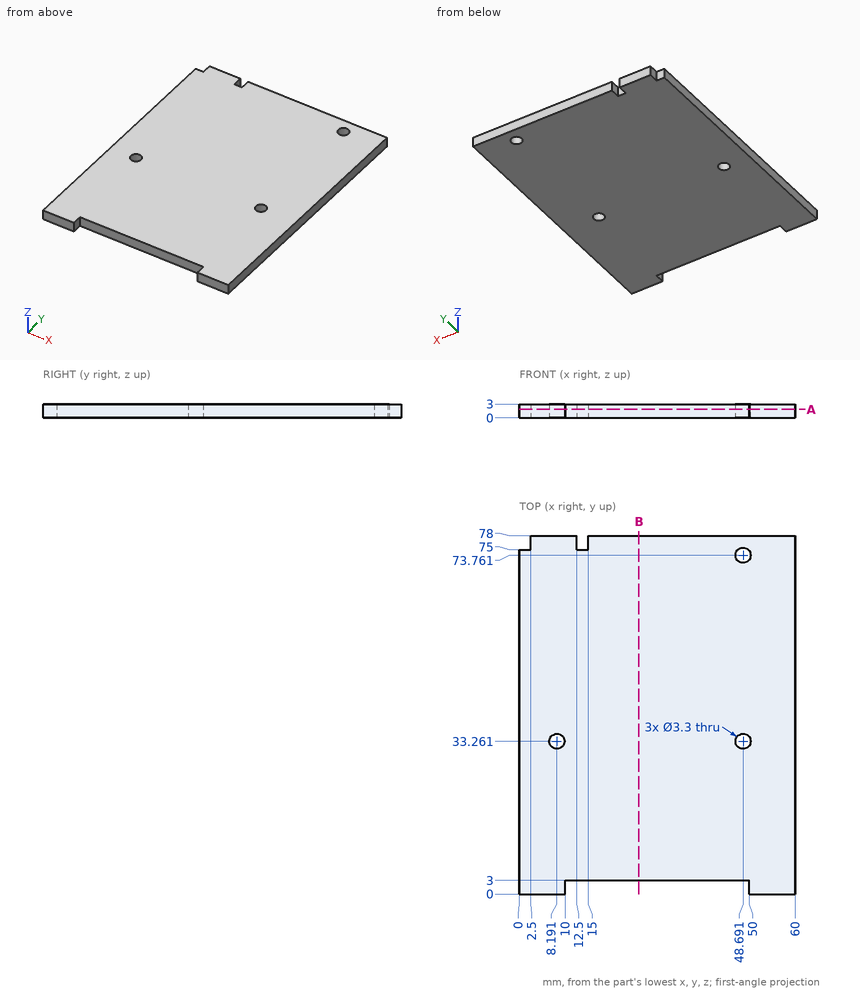
Job drawing, mm, ordinate dimensions from the low corner. One solid piece. Round coordinates to 2 decimals unless told otherwise and drop trailing zeros. Loops run counter-clockwise (first coordinate to the right, second up) from the corner with the lowest first, then second, coordinate; pieces in that order, holes last. Notation, with made-up numbers: (75, 19.5) -> (101, 19.5) arc R8 cw to (101, 33.5) -> close; hole circle Ø5 at (-21.5, 19.5). An arc over 180 degrees is marked (long way). One line per item, written item: value. Start each with the question number.
Q1. Cut at B-B on x = 26. List the corners of the cut face in (y, z).
Q2. Cut at A-A on z = 1.85. List the corners of the cut face in (x, y), plus the area to 3 significant figures.
Q3. Drop flat-ended pins along their axis: pin 1 Ø0.9 at (y, z) = (77, 1.5) entering from -X; pin 2 Ø1 at (y, z) = (30.5, 1.5) entering from -X; pin 3 Ø1.5 at (x, z) = (27, 2) entering from -Y; pin 4 Ø0.8 at (x, z) = (14, 1) entering from +Y. Give the stop position or say it passes through.
Q4. Probe line 1 along Y through (x, z) = (34, 0.3). List the from-to ranges inside material, lowest first.
Computed:
1. outline: (3, 0) -> (78, 0) -> (78, 3) -> (3, 3) -> close
2. outline: (0, 0) -> (10, 0) -> (10, 3) -> (50, 3) -> (50, 0) -> (60, 0) -> (60, 78) -> (15, 78) -> (15, 75) -> (12.5, 75) -> (12.5, 78) -> (2.5, 78) -> (2.5, 75) -> (0, 75) -> close; hole circle Ø3.3 at (8.19, 33.26); hole circle Ø3.3 at (48.69, 33.26); hole circle Ø3.3 at (48.69, 73.76)
2. area: 4,520 mm²
3. pin 1: x = 2.5
3. pin 2: x = 0
3. pin 3: y = 3
3. pin 4: y = 75
4. line 1: 3 to 78
